from build123d import *

# Parameters (mm, degrees)
F0_W     = 25.4
F0_H     = 25.4
F0_W_2   = 19.05
F0_H_2   = 19.05
F1_DEPTH = 203.2
F3_DEPTH = 25.401


with BuildPart() as f1:
    # F0 (on Front) → F1 (new body)
    with BuildSketch(Plane.XZ):
        Rectangle(F0_W, F0_H)
        Rectangle(F0_W_2, F0_H_2, mode=Mode.SUBTRACT)
    extrude(amount=F1_DEPTH)

    # F2 (on face) → F3 (cut, through all)
    with BuildSketch(Plane.YZ.offset(12.7)):
        Polygon((-159.205909, -12.7), (-203.2, 12.7), (-203.2, -12.7), align=None)
        Polygon((0, -12.7), (0, 12.7), (-14.664697, -12.7), align=None)
    extrude(amount=-F3_DEPTH, mode=Mode.SUBTRACT)


solid = f1.part
Could you check a few things on this model? Use its own coordinates, in mm. A direction names the side the tool comes from. Give positions to 0.01 mm unless a question says otherwise; leave off trailing zeros. Order: outer loops, then holes, each group sorted by start corner. A loop starts at its lowest first (then second) coordinate and runs counter-clockwise, first axis right, second up.
Item 1: For faces 4 (the face through (12.7, -100, 0)), 5 (the face through (9.525, -98, 0)), which set-ups out of +Z, -Z, +X, -X, +Y, -Y let a thin tool reach every point of the face, with its end or its side?
Item 2: If we mould it in two halves opening along Z, with no side actions, what happens to faces 1 (the face through (-9.525, -98, 0)), 2 (the face through (-12.7, -100, 0)), 3 (the face through (0, -86, -12.7))? For each: pulls with the +Z half, pulls with the -Z half, needs draft (parallel to the pull), parting line crosses it, or undercut.
Item 3: If we section it at D-D, the plane y = -190: Write out the boundary of the cut face in (x, z) (3 decimals), plus the area to 3 significant figures.
Item 4: If we section it at C-C, the plane z = -4.5: Write out the boundary of the cut face in (x, y) (3 decimals).
Item 5: If we section it at A-A, the plane x = -7.75: Write out the boundary of the cut face in (y, z) (3 decimals), plus the area to 3 significant figures.
Item 6: I'm going to push flat-ended pins straight in: pin 1 (2 mm diameter, centred on x = -1.5, z = 9.5, fed in from +Y); pin 2 (4 mm diameter, centred on x = 4, y = -180.5, fed in from -Z) (3 decimals). Where does each tip first touch, or does it pass through?
Item 7: If we section it at B-B, the plane y = -123: Write out the boundary of the cut face in (x, z) (3 decimals), plus the area to 3 significant figures.
Item 8: I need wall thicknesses on line 1 (X direction, y = -27, z = -6.5) (3 decimals); line 2 (Z direction, x = 9, y = -179) (3 decimals). Which ranges of each line are inside material? Lowest first, please.
Values:
1. face 4: +Z, -Z, +X, +Y, -Y
1. face 5: +Y, -Y
2. face 1: undercut
2. face 2: needs draft
2. face 3: pulls with the -Z half
3. outline: (-12.7, 5.079) - (-9.525, 5.079) - (-9.525, 9.525) - (9.525, 9.525) - (9.525, 5.079) - (12.7, 5.079) - (12.7, 12.7) - (-12.7, 12.7) - close
3. area: 109 mm2
4. outline: (-12.7, -173.409) - (-9.525, -173.409) - (-9.525, -9.93) - (-12.7, -9.93) - close; (9.525, -173.409) - (12.7, -173.409) - (12.7, -9.93) - (9.525, -9.93) - close
5. outline: (-203.2, 12.7) - (-197.701, 9.525) - (-1.833, 9.525) - (0, 12.7) - close; (-164.705, -9.525) - (-159.206, -12.7) - (-14.665, -12.7) - (-12.832, -9.525) - close
5. area: 1,100 mm2
6. pin 1: stops at y = -1.27
6. pin 2: stops at z = 9.525
7. outline: (-12.7, -12.7) - (12.7, -12.7) - (12.7, 12.7) - (-12.7, 12.7) - close; hole (-9.525, -9.525) - (9.525, -9.525) - (9.525, 9.525) - (-9.525, 9.525) - close
7. area: 282 mm2
8. line 1: x = -12.7 to -9.525, 9.525 to 12.7
8. line 2: z = 9.525 to 12.7
